Part model, mm, in its own coordinate system. Face numbers are marked on the shaded views. Round coordinates to 2 decimals unless told otherwise and drop trailing zeros. Order: outer loops, then holes, each group sorted by start corner. A loop starts at its lowest first (then second) coordinate and runs counter-clockwise, first axis right, second up. Notation, with made-up numbers: (31, 57) - (46, 57) arc R28 cw to (46, 83) - close; hole circle Ø9 at (68.5, 48.5). An arc over 180 degrees is marked (long way). Answer as a JSON object with one key per item and string values.
```python
from build123d import *

# Parameters (mm, degrees)
SKETCH1_R           = 2.5
BOSS_EXTRUDE1_DEPTH = 5


with BuildPart() as part:
    # Sketch1 → Boss-Extrude1 (new body)
    with BuildSketch(Plane(origin=(0, 0, 0), x_dir=(0, 0, -1), z_dir=(1, 0, 0))):
        Polygon((8, -10), (-8, -10), (-6, 4.765251939), (6, 4.765251939), align=None)
        Circle(SKETCH1_R, mode=Mode.SUBTRACT)
    extrude(amount=BOSS_EXTRUDE1_DEPTH)


solid = part.part
```
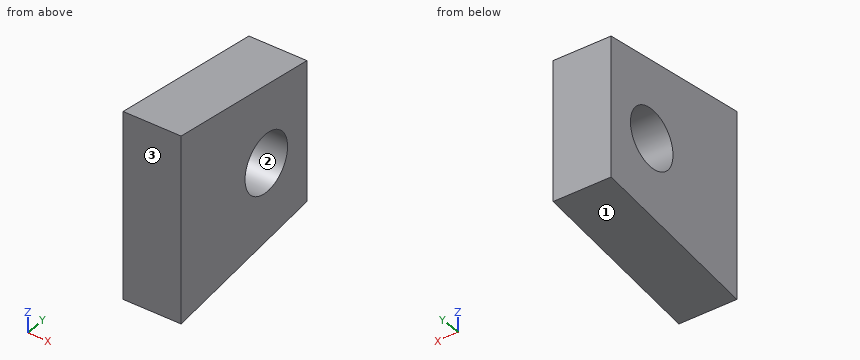
Item 1: Cut at C-C (y = 0). Write the cut outline in (x, z).
Taken from the geometry:
{"outline": "(0, -6.65) - (5, -6.65) - (5, -2.5) - (0, -2.5) - close; (0, 2.5) - (5, 2.5) - (5, 6.65) - (0, 6.65) - close"}
Item 2: Probe L1, parallel to Y at x = 2.55, z = 0; L2, parallel to Z at x = 0.65, y = 2.25; L3, parallel to Z at x = 2, y = -2. List the from-to ranges inside material, lowest first. Write a range as from..to.
Taken from the geometry:
{"L1": "-10..-2.5, 2.5..4.77", "L2": "-6.34..-1.09, 1.09..6.34", "L3": "-6.92..-1.5, 1.5..6.92"}
Item 3: Cut at B-B (z = 0). Write the cut outline in (x, y), plus the area to 3 significant figures.
Taken from the geometry:
{"outline": "(0, -10) - (5, -10) - (5, -2.5) - (0, -2.5) - close; (0, 2.5) - (5, 2.5) - (5, 4.77) - (0, 4.77) - close", "area": "48.8 mm2"}
Item 4: Drop flat-ended pins along their axis: P1, Ø1, axis at x = 3, y = 1.5, coming from the -Z side; P2, Ø2, axis at y = -6, z = -4, coming from the -X side. Give the stop position or say it passes through.
Taken from the geometry:
{"P1": "z = -6.51", "P2": "x = 0"}
Item 5: Two-plate mould, pull along Z, no slides. Class the marked faces 1, 2 and 3: pulls with the +Z half, pulls with the -Z half, needs draft (parallel to the pull), parting line crosses it, or undercut.
Taken from the geometry:
{"face 1": "pulls with the -Z half", "face 2": "undercut", "face 3": "needs draft"}
Item 6: Cut at A-A (x = 1.5). Write the cut outline in (y, z), plus the area to 3 significant figures.
Taken from the geometry:
{"outline": "(-10, -8) - (4.77, -6) - (4.77, 6) - (-10, 8) - close; hole circle Ø5 at (0, 0)", "area": "187 mm2"}
Item 7: Cut at D-D (y = 3). Write the cut outline in (x, z), plus the area to 3 significant figures.
Taken from the geometry:
{"outline": "(0, -6.24) - (5, -6.24) - (5, 6.24) - (0, 6.24) - close", "area": "62.4 mm2"}
